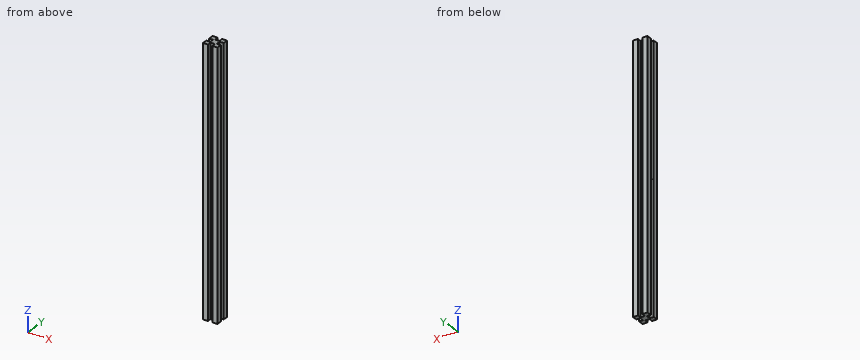
```python
from build123d import *

# Parameters (mm, degrees)
F1_DEPTH = 360
F2_R     = 3
F3_DEPTH = 25


with BuildPart() as f1:
    # F0 (on Top) → F1 (new body)
    with BuildSketch(Plane.XY):
        Polygon((0, 7), (0, 0), (7, 0), (7, 5.5), (13, 5.5), (13, 0), (20, 0), (20, 7), (14.5, 7), (14.5, 13), (20, 13), (20, 20), (13, 20), (13, 14.5), (7, 14.5), (7, 20), (0, 20), (0, 13), (5.5, 13), (5.5, 7), align=None)
    extrude(amount=F1_DEPTH)

    # F2 (on face) → F3 (cut)
    with BuildSketch(Plane.YZ.offset(14.5)):
        with Locations((9.993159, 180)):
            Circle(F2_R)
    extrude(amount=-F3_DEPTH, mode=Mode.SUBTRACT)


solid = f1.part
```
The listing builds one solid part. Answer for the finished solid, in the listing's coordinates (mm). Round coordinates to 2 decimals unless told otherwise and drop trailing zeros. Write each loop counter-clockwise with the first axis right and the second up, starting at its lowest first coordinate (ties: lowest second). Pieces come first, ordered by that corner, then holes. Notation, with made-up numbers: (9.5, -24) -> (51.5, -24) arc R18 ccw to (51.5, -16) -> close; hole circle Ø7 at (9, 76). An arc over 180 degrees is marked (long way). Use CSV: the item, a comma, the result in double quotes. Start each with the question number.
(1) Section A-A on z = 76.5 is taken. Give the vertices of the cut face in (x, y), then the cut area to 3 significant figures.
(2) This flat-tipped pin is pushed along its axis until it touches: pin 1 (1.8 mm diameter, centred on y = 9, z = 144, fed in from +X). Where does it stop, or does it pass through?
(3) Section B-B on x = 10 is taken. Give the vertices of the cut face in (y, z).
(4) Consider L1, parallel to X at y = 3.75, z = 105.5; L2, parallel to Y at x = 7.25, z = 180. Determine where each line is inside the solid, lowest interval first. Write a range as from..to.
A:
1,outline,"(0, 0) -> (7, 0) -> (7, 5.5) -> (13, 5.5) -> (13, 0) -> (20, 0) -> (20, 7) -> (14.5, 7) -> (14.5, 13) -> (20, 13) -> (20, 20) -> (13, 20) -> (13, 14.5) -> (7, 14.5) -> (7, 20) -> (0, 20) -> (0, 13) -> (5.5, 13) -> (5.5, 7) -> (0, 7) -> close"
1,area,"268 mm²"
2,pin 1,"stops at x = 14.5"
3,outline,"(5.5, 0) -> (14.5, 0) -> (14.5, 360) -> (5.5, 360) -> close; hole circle Ø6 at (9.99, 180)"
4,L1,"x = 0..7, 13..20"
4,L2,"y = 5.5..6.99, 12.99..14.5"
